Could you check a few things on this drawing? It's one solid part, dimensions in mm from its lowest x, y, z. A direction names the side the tool comes from. Give positions to 0.01 mm unless a question says otherwise; leave off trailing zeros. Order: outer loops, then holes, each group sorted by start corner. A loop starts at its lowest first (then second) coordinate and runs counter-clockwise, first axis right, second up.
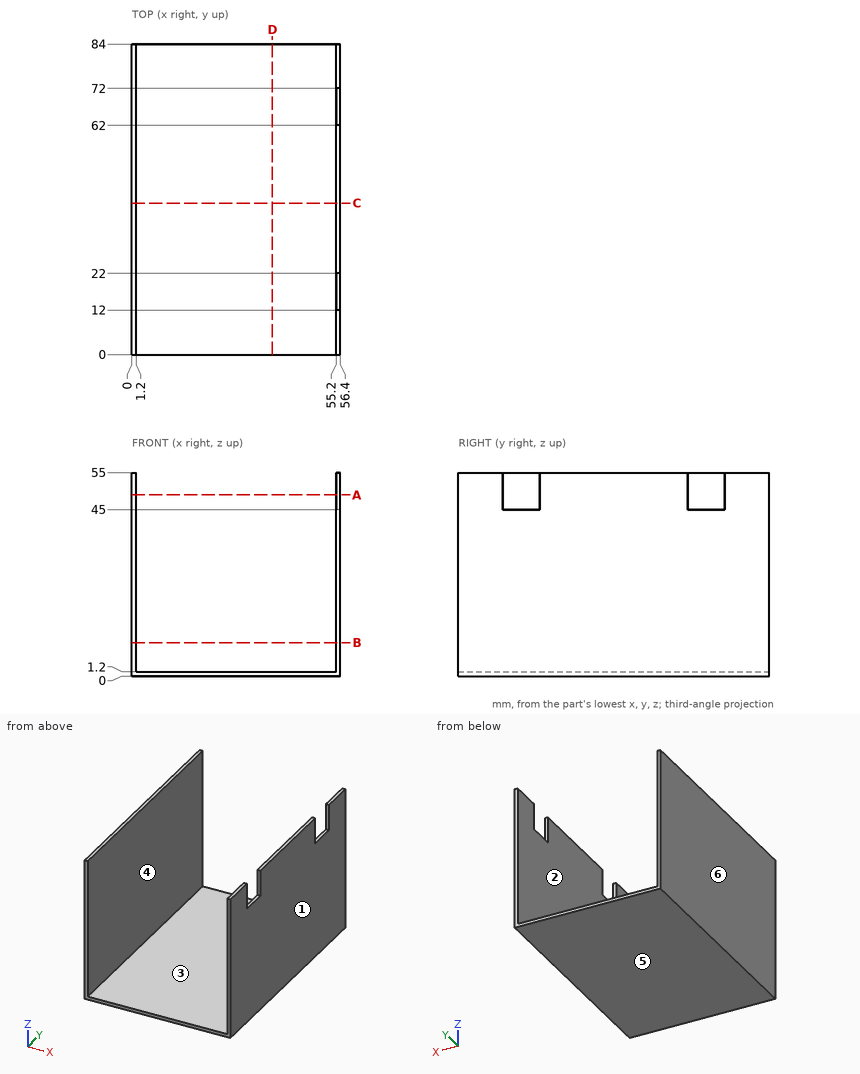
Q1. If we section it at A-A on z = 49: List the corners of the cut face in (x, y) for me, plus the area to 3 significant figures.
Filled sheet:
outline: (0, 0) - (1.2, 0) - (1.2, 84) - (0, 84) - close; (55.2, 0) - (56.4, 0) - (56.4, 12) - (55.2, 12) - close; (55.2, 22) - (56.4, 22) - (56.4, 62) - (55.2, 62) - close; (55.2, 72) - (56.4, 72) - (56.4, 84) - (55.2, 84) - close
area: 178 mm2
Q2. If we section it at D-D on x = 38: List the corners of the cut face in (y, z) for me.
Filled sheet:
outline: (0, 0) - (84, 0) - (84, 1.2) - (0, 1.2) - close
Q3. For the marked faces 1 and 2, which set-ups out of +Z, -Z, +X, -X, +Y, -Y let a thin tool reach every point of the face, with its end or its side?
Filled sheet:
face 1: +Z, -Z, +X, +Y, -Y
face 2: +Z, +Y, -Y
Q4. If we section it at C-C on y = 41: List the corners of the cut face in (x, z) for me, plus the area to 3 significant figures.
Filled sheet:
outline: (0, 0) - (56.4, 0) - (56.4, 55) - (55.2, 55) - (55.2, 1.2) - (1.2, 1.2) - (1.2, 55) - (0, 55) - close
area: 197 mm2
Q5. I need wall thicknesses on L1, parallel to X at y = 39, z = 38.5; L2, parallel to Z at x = 52, y = 39. Which ranges of each line are inside material? Lowest first, please.
Filled sheet:
L1: x = 0 to 1.2, 55.2 to 56.4
L2: z = 0 to 1.2
Q6. I'm going to push flat-ended pins straight in: P1, Ø1.5, axis at x = 16, y = 25.5, coming from the +Z side; P2, Ø1, axis at x = 55.5, y = 16, coming from the +Z side. Where does each tip first touch, or does it pass through?
Filled sheet:
P1: stops at z = 1.2
P2: stops at z = 45
Q7. Thinking about a two-plate mould opening in X: for the marked faces 3, 4, 5 and 6, which applies, released by +X, released by -X, zero draft, split by the parting line, or undercut?
Filled sheet:
face 3: undercut
face 4: undercut
face 5: zero draft
face 6: released by -X
Q8. If we section it at B-B on z = 9: List the corners of the cut face in (x, y) for me.
Filled sheet:
outline: (0, 0) - (1.2, 0) - (1.2, 84) - (0, 84) - close; (55.2, 0) - (56.4, 0) - (56.4, 84) - (55.2, 84) - close
